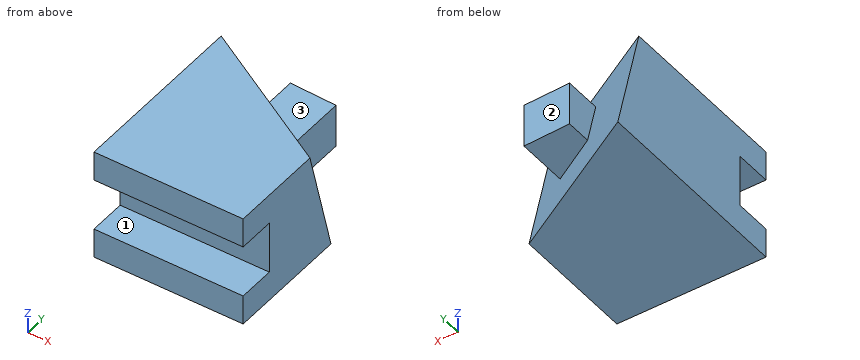
```python
from build123d import *

# Parameters (mm, degrees)
SKETCH1_W                = 60
SKETCH1_H                = 45
BOSS_EXTRUDE1_DEPTH      = 85
SKETCH2_W                = 21
SKETCH2_H                = 15
CUT_EXTRUDE1_DEPTH       = 85
CUT_EXTRUDE7_DEPTH       = 53
CUT_EXTRUDE9_DEPTH       = 42
CUT_EXTRUDE10_DEPTH      = 42
BOSS_EXTRUDE6_DEPTH      = 15
BOSS_EXTRUDE6_DEPTH_BACK = 15


with BuildPart() as part:
    # Sketch1 → Boss-Extrude1 (new body)
    with BuildSketch(Plane(origin=(0, 0, 0), x_dir=(1, 0, 0), z_dir=(0, 1, 0))):
        with Locations((30, 22.5)):
            Rectangle(SKETCH1_W, SKETCH1_H)
    extrude(amount=BOSS_EXTRUDE1_DEPTH)

    # Sketch2 → Cut-Extrude1 (cut)
    with BuildSketch(Plane(origin=(60, 0, 0), x_dir=(0, 0, -1), z_dir=(1, 0, 0))):
        with Locations((22.5, 7.5)):
            Rectangle(SKETCH2_W, SKETCH2_H)
    extrude(amount=-CUT_EXTRUDE1_DEPTH, mode=Mode.SUBTRACT)

    # Sketch10 → Cut-Extrude7 (cut)
    with BuildSketch(Plane.XY):
        Polygon((0, 85), (60, 50.358983849), (60, 85), align=None)
    extrude(amount=-CUT_EXTRUDE7_DEPTH, mode=Mode.SUBTRACT)

    # Sketch16 → Cut-Extrude9 (cut)
    with BuildSketch(Plane.ZY):
        Polygon((-45, 85), (0, 72.942286341), (0, 85), align=None)
    extrude(amount=-CUT_EXTRUDE9_DEPTH, mode=Mode.SUBTRACT)

    # Sketch17 → Cut-Extrude10 (cut)
    with BuildSketch(Plane(origin=(29.971067136, 51.911411037, 13.909620665), x_dir=(0.873369362, -0.470462359, -0.126060009), z_dir=(0.487058474, 0.843610023, 0.226044624))):
        Polygon((34.382855821, 56.500526295), (34.382855821, 9.913098177), (-34.316600088, 18.878852898), (-34.316600088, 65.466281017), align=None)
    extrude(amount=CUT_EXTRUDE10_DEPTH, mode=Mode.SUBTRACT)

    # Sketch38 → Boss-Extrude6 (add, two sides)
    with BuildSketch(Plane(origin=(0, 60.290929389, 0), x_dir=(-1, 0, 0), z_dir=(0, -1, 0))) as boss_extrude6_sk:
        Polygon((-26.20108087, 9.239976128), (-44.541837479, 10.004497867), (-44.541837479, 27.465894941), (-26.20108087, 26.701373203), align=None)
    extrude(amount=BOSS_EXTRUDE6_DEPTH)
    extrude(boss_extrude6_sk.sketch, amount=-BOSS_EXTRUDE6_DEPTH_BACK)


solid = part.part
```
Source: CAD feature listing. Evaluate the final solid. Frame: model axes, mm. Face numbers are marked on the shaded views. A direction names the side the tool comes from. Coordinates: 2 decimals unless noted, no trailing zeros. Loops run counter-clockwise (first coordinate to the right, second up) from the corner with the lowest first, then second, coordinate; pieces in that order, holes last. Notation, with made-up numbers: (-8, 50.25) - (-4, 50.25) arc R28 cw to (-4, 71.25) - close; hole circle Ø8 at (-20.5, -28). An arc over 180 degrees is marked (long way). Answer as CSV lines item,"result".
1. Section D-D (y = 66.5). Return loops of the section in (x, z), then the cut area to 3 significant figures.
Established:
outline,"(0, -45) - (32.04, -45) - (11.16, 0) - (0, 0) - close; (26.2, -26.7) - (44.54, -27.47) - (44.54, -10) - (26.2, -9.24) - close"
area,"1,290 mm2"
2. Reachability of the marked faces 1, 2 and 3 from +Z, -Z, +X, -X, +Y, -Y: full face, straight path, thin tool, end or side. Return the list, or none.
Established:
face 1,"+X, -X, -Y"
face 2,"+Z, -Z, +X, +Y"
face 3,"+Z, +X, +Y"
3. Section B-B (z = -18.5). Return loops of the section in (x, y), then the cut area to 3 significant figures.
Established:
outline,"(0, 15) - (60, 15) - (60, 43.26) - (44.54, 52.18) - (44.54, 75.29) - (26.2, 75.29) - (26.2, 62.77) - (0, 77.9) - close"
area,"3,060 mm2"
4. Section A-A (y = 12). Return loops of the section in (x, z), then the cut area to 3 significant figures.
Established:
outline,"(0, -45) - (60, -45) - (60, -33) - (0, -33) - close; (0, -12) - (60, -12) - (60, 0) - (0, 0) - close"
area,"1,440 mm2"
5. Contact query for flat-ended pins moving along their axis: pin 1 (3 mm diameter, centred on x = 40.5, z = -25, fed in from +Y); pin 2 (2 mm diameter, centred on x = 6.5, z = -31, fed in from -Y); pin 3 (8.5 mm diameter, centred on y = 58.5, z = -22, fed in from +X). Output: stop coordinate, or through.
Established:
pin 1,"stops at y = 75.29"
pin 2,"stops at y = 15"
pin 3,"stops at x = 44.54"
6. Ray query, line 1 (Z direction, x = 43, y = 7); line 2 (X direction, y = 72, z = -26); line 3 (X direction, y = 71, z = -13). Return the intervals inside material, ascending.
Established:
line 1,"z = -45 to -33, -12 to 0"
line 2,"x = 0 to 13.7, 26.2 to 44.54"
line 3,"x = 0 to 9.4, 26.2 to 44.54"
7. Section C-C (x = 48.5). Return loops of the section in (y, z), then the cut area to 3 significant figures.
Established:
outline,"(0, -45) - (57, -45) - (44.94, 0) - (0, 0) - (0, -12) - (15, -12) - (15, -33) - (0, -33) - close"
area,"1,980 mm2"
